Check sheet for the drawn part. Datum: minimum x, y, z corner. Units: mm. Round coordinates to 2 decimals unless told otherwise and drop trailing zeros. Write each loop counter-clockwise with the first axis right and the second up, starting at its lowest first coordinate (ties: lowest second). Pieces come first, ordered by that corner, then holes. Notation, with made-up numbers: M 16,86.5 L 73,86.5 A26 ccw 73,104.5 Z; hole C 84.25,6 d5. An arc over 180 degrees is marked long. Put each result on its own line as item: value.
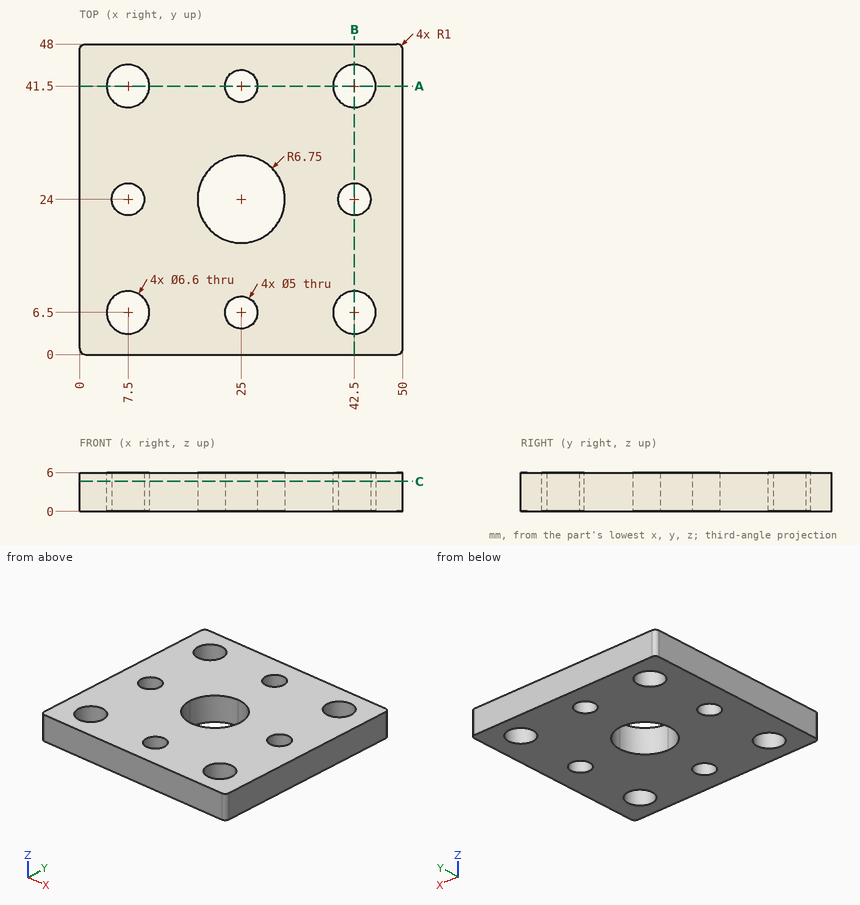
1. Cross-section at B-B (x = 42.5). Enter the section's corners in (y, z), then the cut area to 3 significant figures.
Computed values:
outline: M 0,0 L 3.2,0 L 3.2,6 L 0,6 Z; M 9.8,0 L 21.5,0 L 21.5,6 L 9.8,6 Z; M 26.5,0 L 38.2,0 L 38.2,6 L 26.5,6 Z; M 44.8,0 L 48,0 L 48,6 L 44.8,6 Z
area: 179 mm2
2. Cross-section at A-A (y = 41.5). Enter the section's corners in (x, z), then the cut area to 3 significant figures.
Computed values:
outline: M 0,0 L 4.2,0 L 4.2,6 L 0,6 Z; M 10.8,0 L 22.5,0 L 22.5,6 L 10.8,6 Z; M 27.5,0 L 39.2,0 L 39.2,6 L 27.5,6 Z; M 45.8,0 L 50,0 L 50,6 L 45.8,6 Z
area: 191 mm2
3. Scan lines: probe 1 along Y at (x, z) = (42.5, 2.75); probe 2 along Y at (x, z) = (24, 1.7); probe 3 along X at (y, z) = (38.5, 5.05). Record each from-to range of solid material in increasing order.
Computed values:
probe 1: y = 0 to 3.2, 9.8 to 21.5, 26.5 to 38.2, 44.8 to 48
probe 2: y = 0 to 4.21, 8.79 to 17.32, 30.68 to 39.21, 43.79 to 48
probe 3: x = 0 to 6.13, 8.87 to 41.13, 43.87 to 50
4. Cross-section at C-C (z = 4.65). Count the separate pieces of the cut face and the enclosed holes in it, then the cut area to 3 significant figures.
Computed values:
separate pieces: 1
enclosed holes: 9
area: 2,040 mm2
5. Depth check by flat-ended pin: pin 1 Ø3 at (x, y) = (25, 41.5) entering from -Z. Enter the tip coordinate at first touch or a pass-through.
Computed values:
pin 1: passes through
